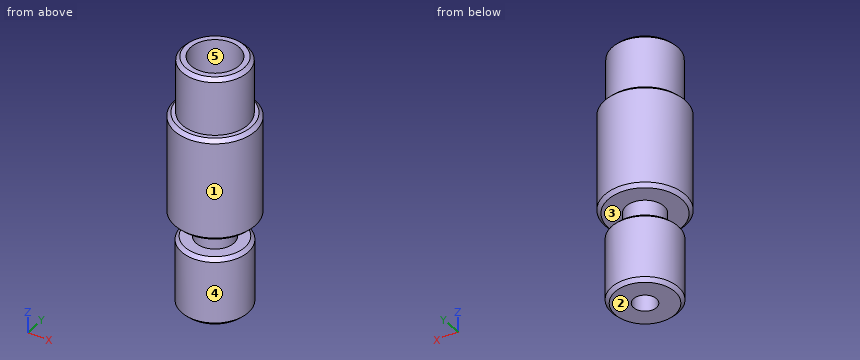
from build123d import *

# Parameters (mm, degrees)
F2_SIZE = 0.3


with BuildPart() as f1:
    # F0 (on Front) → F1 (revolve)
    with BuildSketch(Plane.XZ):
        Polygon((2.85, 22), (2.1, 22), (2.1, 9), (1, 8.339053), (1, 0), (2.9, 0), (2.9, 6), (1.65, 6), (1.65, 8), (3.5, 8), (3.5, 17), (2.85, 17), align=None)
    revolve(axis=Axis((0, 0, 11), (0, 0, 1)))

    # F2
    f2_edges = [f1.edges().sort_by_distance(p)[0] for p in [
        (-2.85, 0, 22),
        (-3.5, 0, 17),
        (-3.5, 0, 8),
        (-2.9, 0, 6),
        (-2.9, 0, 0),
    ]]
    chamfer(f2_edges, length=F2_SIZE)


solid = f1.part
The listing builds one solid part. Answer for the finished solid, in the listing's coordinates (mm). Face numbers are marked on the shaded views. A direction names the side the tool comes from. Give positions to 0.01 mm unless a question says otherwise; leave off trailing zeros. Write each loop counter-clockwise with the first axis right and the second up, starting at its lowest first coordinate (ties: lowest second). Pieces come first, ordered by that corner, then holes.
1) Section B-B (z = 13.25) is taken. Write down the section's boundary in (x, y), and give its area (3 significant figures).
2) For a pull along Z with two mould halves and no side action, classify the marked faces 1, 2 and 3 as pulls with the +Z half, pulls with the -Z half, needs draft (parallel to the pull), parting line crosses it, or undercut.
3) A tool of negligible diameter and unlimited length cuts with its end or side. For the marked faces 4 and 5, from which of +Z, -Z, +X, -X, +Y, -Y can it reach the whole face along a straight path? Write none if from no direction.
4) Section C-C (z = 5) is taken. Write down the section's boundary in (x, y), and give its area (3 significant figures).
5) Find the intervals of material crossed by L1, parallel to Y at x = 0, z = 18.5; L2, parallel to Y at x = 0, z = 6.5; L3, parallel to Z at x = 1.25, y = 1.75, in increasing order.
6) Given P1, Ø1.9, axis at x = 0, y = 1, coming from the +Z side; P2, Ø3, axis at x = 0, y = 0, coming from the +Z side; P3, Ø2, axis at y = -2.5, z = 6, coming from the -X side, each flat-ended and moving along its own axis, determine where each tip first touches the part or whether it passes through.
Response:
1. outline: circle Ø7 at (0, 0); hole circle Ø4.2 at (0, 0)
1. area: 24.6 mm2
2. face 1: needs draft
2. face 2: pulls with the -Z half
2. face 3: undercut
3. face 4: -Z
3. face 5: +Z
4. outline: circle Ø5.8 at (0, 0); hole circle Ø2 at (0, 0)
4. area: 23.3 mm2
5. L1: y = -2.85 to -2.1, 2.1 to 2.85
5. L2: y = -1.65 to -1, 1 to 1.65
5. L3: z = 0 to 6, 8 to 22
6. P1: stops at z = 8.91
6. P2: stops at z = 8.64
6. P3: stops at x = -2.45
